The listing builds one solid part. Answer for the finished solid, in the listing's coordinates (mm). Give positions to 0.01 mm unless a question says otherwise; leave off trailing zeros. Write each loop counter-clockwise with the first axis right and the second up, starting at its lowest first coordinate (ties: lowest second). Pieces come first, ordered by that corner, then holes. Notation, with made-up numbers: (74.5, -18) - (83.5, -18) arc R16 ccw to (83.5, -12) - close; hole circle Ø4 at (36, 64.5). An arc over 180 degrees is marked (long way). Answer as CSV lines item,"result". Start each with the question number.
(1) Find section C-C (z = 9). Write down the section's boundary in (x, y).
(2) Straight lines are drawn through the part: probe 1 along Y at (x, z) = (0, -5); probe 2 along X at (y, z) = (1.75, -10); probe 3 along Y at (x, z) = (-1.25, 4). For each, find the intervals that lie inside material, in ascending order.
(3) Find section B-B (y = 0). Write down the section's boundary in (x, z) (3 decimals), then the cut area to 3 significant figures.
(4) Find section D-D (y = 3). Write down the section's boundary in (x, z) (3 decimals), then the cut area to 3 significant figures.
(5) For a pull along X with two mould halves and no side action, classify faces 1 (the face through (-11.43, -0.05, 0.22)), 2 (the face through (2.032, 0, 0)), 3 (the face through (-2.665, -0.091, 0.222)), 4 (the face through (5.591, -3.634, 0.222)) as pulls with the +X half, pulls with the -X half, needs draft (parallel to the pull), parting line crosses it, or undercut.
(6) Each of these flat-tipped pins is pushed along its axis until it touches: pin 1 Ø5 at (y, z) = (-3.5, 6.5) entering from +X; pin 2 Ø5 at (x, z) = (6.5, 5) entering from +Y. Where does it stop, or does it pass through?
(7) Find section A-A (x = 0). Write down the section's boundary in (y, z) (3 decimals), then the cut area to 3 significant figures.
from build123d import *

# Parameters (mm, degrees)
BOSS_EXTRUDE1_DEPTH = 15.875


with BuildPart() as part:
    # Sketch1 → Boss-Extrude1 (new, symmetric)
    with BuildSketch(Plane.XY):
        with BuildLine():
            Line((-9.615714286, 2.434119713), (-1.451428571, 4.868239425))
            ThreePointArc((-1.451428571, 4.868239425), (0, 5.08), (1.451428571, 4.868239425))
            Line((1.451428571, 4.868239425), (9.615714286, 2.434119713))
            ThreePointArc((9.615714286, 2.434119713), (11.43, 0), (9.615714286, -2.434119713))
            Line((9.615714286, -2.434119713), (1.451428571, -4.868239425))
            ThreePointArc((1.451428571, -4.868239425), (0, -5.08), (-1.451428571, -4.868239425))
            Line((-1.451428571, -4.868239425), (-9.615714286, -2.434119713))
            ThreePointArc((-9.615714286, -2.434119713), (-11.43, 0), (-9.615714286, 2.434119713))
        make_face()
        with BuildLine():
            Line((2.032, 1.727386755), (2.032, -1.727386755))
            ThreePointArc((2.032, -1.727386755), (-2.667, 0), (2.032, 1.727386755))
        make_face(mode=Mode.SUBTRACT)
    extrude(amount=BOSS_EXTRUDE1_DEPTH, both=True)


solid = part.part
Result set:
1,outline,"(-9.62, -2.43) - (-1.45, -4.87) arc R5.08 ccw to (1.45, -4.87) - (9.62, -2.43) arc R2.54 ccw to (9.62, 2.43) - (1.45, 4.87) arc R5.08 ccw to (-1.45, 4.87) - (-9.62, 2.43) arc R2.54 ccw to start; hole (2.03, -1.73) - (2.03, 1.73) arc R2.67 ccw (long way) to start"
2,probe 1,"-5.08 to -2.67, 2.67 to 5.08"
2,probe 2,"-10.73 to -2.01, 2.01 to 10.73"
2,probe 3,"-4.92 to -2.36, 2.36 to 4.92"
3,outline,"(-11.43, -15.875) - (-2.667, -15.875) - (-2.667, 15.875) - (-11.43, 15.875) - close; (2.032, -15.875) - (11.43, -15.875) - (11.43, 15.875) - (2.032, 15.875) - close"
3,area,"577 mm^2"
4,outline,"(-7.718, -15.875) - (7.718, -15.875) - (7.718, 15.875) - (-7.718, 15.875) - close"
4,area,"490 mm^2"
5,face 1,"pulls with the -X half"
5,face 2,"undercut"
5,face 3,"undercut"
5,face 4,"pulls with the +X half"
6,pin 1,"x = 11.22"
6,pin 2,"y = 4.11"
7,outline,"(-5.08, -15.875) - (-2.667, -15.875) - (-2.667, 15.875) - (-5.08, 15.875) - close; (2.667, -15.875) - (5.08, -15.875) - (5.08, 15.875) - (2.667, 15.875) - close"
7,area,"153 mm^2"
